For this review, use the dimensioned drawing (mm, ordinates from the lowest corner) and the shaded views. Give positions to 0.01 mm unless a question says otherwise; leave off trailing zeros. Write each loop counter-clockwise with the first axis right and the second up, starting at its lowest first coordinate (ties: lowest second). Pieces come first, ordered by that corner, then holes. Notation, with made-up numbers: M 29,-18.75 L 37,-18.75 A21 cw 37,-13.75 Z; hole C -3.75,81.25 d9. An arc over 180 degrees is marked long. Answer in a Markdown table with one row per item.
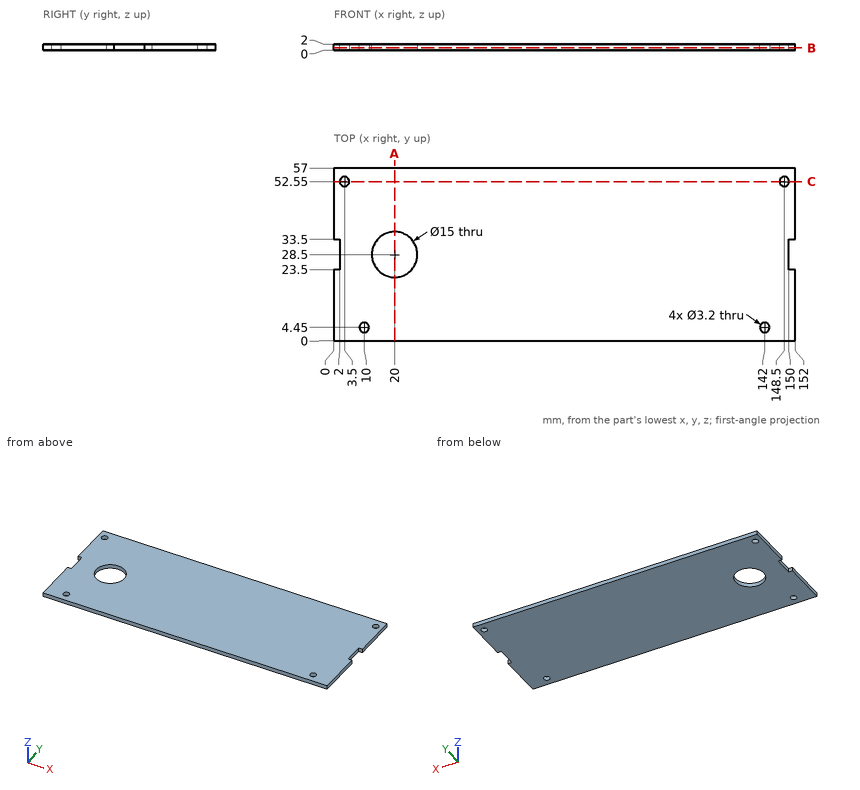
1) Insertion check: P1, Ø1, axis at x = 1.5, z = 1, coming from the -Y side; P2, Ø2.5, axis at x = 142, y = 4.45, coming from the -Z side; P3, Ø0.6, axis at y = 28.5, z = 1, coming from the +X side. Each pin has a flat end and moves straight along its axis. Give the tip position at first contact, or say it passes through.
Geometry says:
| item | result |
|---|---|
| P1 | y = 0 |
| P2 | through |
| P3 | x = 150 |
2) Add section A-A (x = 20). Write out the cut boundary in (y, z), and give its area (3 significant figures).
Geometry says:
| item | result |
|---|---|
| outline | M 0,0 L 21,0 L 21,2 L 0,2 Z; M 36,0 L 57,0 L 57,2 L 36,2 Z |
| area | 84.0 mm^2 |
3) Add section B-B (z = 0.7). Write out the cut boundary in (x, y).
Geometry says:
| item | result |
|---|---|
| outline | M 0,0 L 152,0 L 152,23.5 L 150,23.5 L 150,33.5 L 152,33.5 L 152,57 L 0,57 L 0,33.5 L 2,33.5 L 2,23.5 L 0,23.5 Z; hole C 3.5,52.55 d3.2; hole C 10,4.45 d3.2; hole C 20,28.5 d15; hole C 142,4.45 d3.2; hole C 148.5,52.55 d3.2 |
4) To check wall thickness, follow probe 1 along X at (y, z) = (52.5, 0.45); probe 2 along Y at (x, z) = (20, 1.45); probe 3 along Y at (x, z) = (142, 0.5). State the ranges of each line that lie inside material, in increasing order. Write a range as [from, to].
Geometry says:
| item | result |
|---|---|
| probe 1 | [0, 1.9], [5.1, 146.9], [150.1, 152] |
| probe 2 | [0, 21], [36, 57] |
| probe 3 | [0, 2.85], [6.05, 57] |
5) Add section C-C (y = 52.55). Write out the cut boundary in (x, z).
Geometry says:
| item | result |
|---|---|
| outline | M 0,0 L 1.9,0 L 1.9,2 L 0,2 Z; M 5.1,0 L 146.9,0 L 146.9,2 L 5.1,2 Z; M 150.1,0 L 152,0 L 152,2 L 150.1,2 Z |
